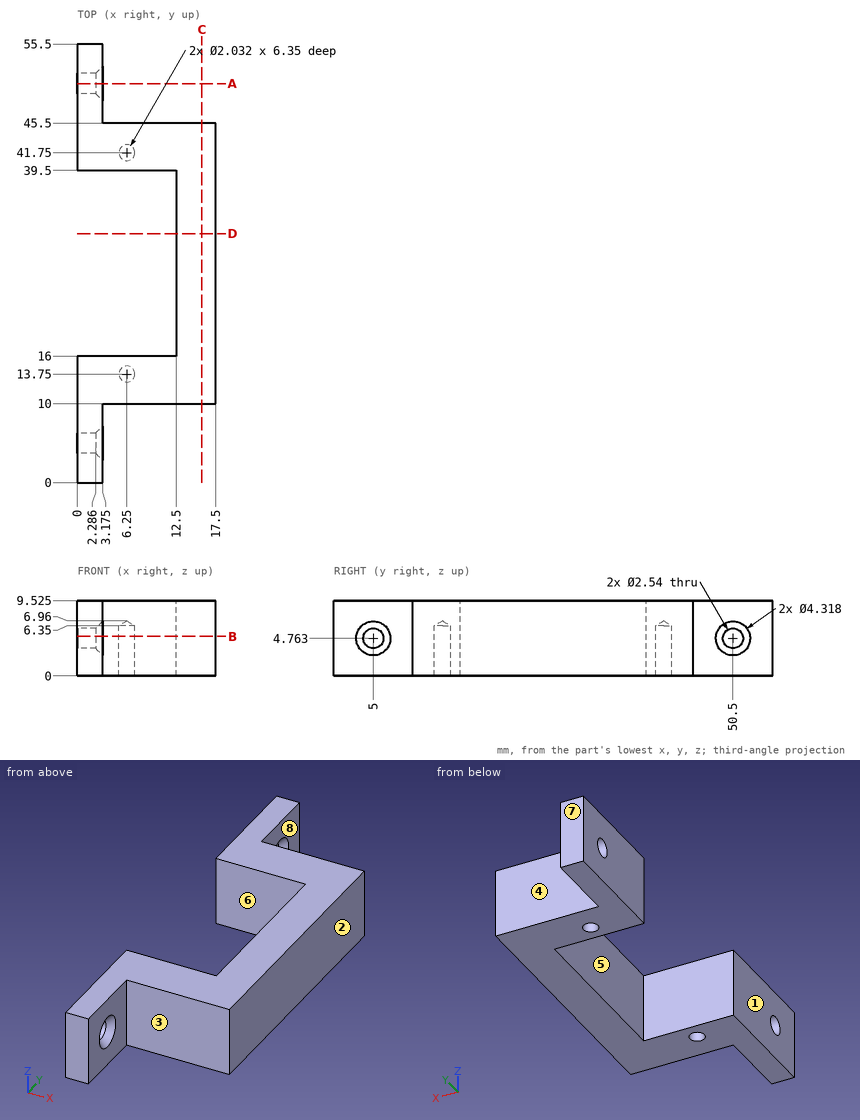
Part print with two shaded views. Sizes in mm from the minimum x, y, z corner. A direction names the side the tool comes from. Coordinates: 2 decimals unless noted, no trailing zeros. Write each loop counter-clockwise with the first axis right and the second up, starting at its lowest first coordinate (ties: lowest second). Pieces come first, ordered by that corner, then holes. Notation, with made-up numbers: (70.5, -13.75) - (76.5, -13.75) arc R22 cw to (76.5, -0.75) - close; hole circle Ø6 at (15.25, 81.5). An arc over 180 degrees is marked (long way). Use a Markdown table: item, result. Add a question column.
Item 1: Band-saw the part on C-C, the plane x = 15.75. Write the cut outline in (y, z) (1 decimal), and give its area (3 significant figures).
Item 2: Band-saw the part on B-B, the plane z = 5. Give the number of separate pieces and of enclosed holes in the cut face, and give its area (3 significant figures).
Item 3: 3-axis set-ups, long thin cutter, end or side, ignore diameter. For the marked faces 1, 2, 3, 4 and 5: which of +Z, -Z, +X, -X, +Y, -Y reach the whole face in a straight line?
Item 4: Band-saw the part on A-A, the plane y = 50.5. Write the cut outline in (x, z) (1 decimal).
Item 5: Two-plate mould, pull along Y, no slides. Class the marked faces 6, 7 and 8: pulls with the +Y half, pulls with the -Y half, needs draft (parallel to the pull), parting line crosses it, or undercut.
Item 6: Drill centre lines: line 1 along Y through (x, z) = (6.25, 2.5) (1 decimal); line 2 along Z through (x, y) = (0.85, 50.5) (1 decimal); line 3 along X through (y, z) = (13.75, 1.75) (1 decimal). Where is each one in solid material? Low to high.
Item 7: Band-saw the part on D-D, the plane y = 31.5. Write the cut outline in (x, z) (1 decimal).
Item 8: Drop flat-ended pins along their axis: pin 1 (5 mm diameter, centred on x = 11, z = 6.5, fed in from +Y); pin 2 (1.2 mm diameter, centred on x = 6.25, y = 41.75, fed in from -Z); pin 3 (5 mm diameter, centred on y = 24.5, z = 5.5, fed in from -X). Give the stop position or say it passes through.
A:
| question | item | result |
|---|---|---|
| 1 | outline | (10, 0) - (45.5, 0) - (45.5, 9.5) - (10, 9.5) - close |
| 1 | area | 338 mm² |
| 2 | separate pieces | 3 |
| 2 | enclosed holes | 2 |
| 2 | area | 367 mm² |
| 3 | face 1 | +Z, -Z, -X, +Y, -Y |
| 3 | face 2 | +Z, -Z, +X, +Y, -Y |
| 3 | face 3 | +Z, -Z, +X, -Y |
| 3 | face 4 | +Z, -Z, +X, +Y |
| 3 | face 5 | +Z, -Z, -X |
| 4 | outline | (0, 0) - (3.2, 0) - (3.2, 2.6) - (2.3, 3.5) - (0, 3.5) - close; (0, 6) - (2.3, 6) - (3.2, 6.9) - (3.2, 9.5) - (0, 9.5) - close |
| 5 | face 6 | undercut |
| 5 | face 7 | pulls with the +Y half |
| 5 | face 8 | needs draft |
| 6 | line 1 | y = 10 to 12.7, 14.8 to 16, 39.5 to 40.7, 42.8 to 45.5 |
| 6 | line 2 | z = 0 to 3.5, 6 to 9.5 |
| 6 | line 3 | x = 0 to 5.2, 7.3 to 17.5 |
| 7 | outline | (12.5, 0) - (17.5, 0) - (17.5, 9.5) - (12.5, 9.5) - close |
| 8 | pin 1 | stops at y = 45.5 |
| 8 | pin 2 | stops at z = 6.6 |
| 8 | pin 3 | stops at x = 12.5 |
